from build123d import *

# Parameters (mm, degrees)
SPUR_START             = -44.074195703
SPUR_GEAR_AI_OUTLINE_R = 4.7625
SPUR_GEAR_AI_DEPTH     = 14.605
CUT_EXTRUDE1_DEPTH     = 39.307434666


# Read off the part's stored shape, not the designer's step: spur gear_ai
with BuildPart() as part:
    # spur gear_ai outline → spur gear_ai (new body)
    with BuildSketch(Plane.YZ.offset(SPUR_START)):
        with BuildLine():
            ThreePointArc((12.686684526, 14.250652999), (12.919777657, 14.586350288), (13.140720632, 14.930166051))
            ThreePointArc((13.140720632, 14.930166051), (12.265878987, 16.134593199), (11.016013995, 16.943190851))
            ThreePointArc((11.016013995, 16.943190851), (11.347770551, 17.651104248), (11.613753604, 18.386261921))
            ThreePointArc((11.613753604, 18.386261921), (13.069306498, 18.074238793), (14.539571561, 18.307290937))
            ThreePointArc((14.539571561, 18.307290937), (14.626455743, 18.70663567), (14.699007839, 19.108831233))
            ThreePointArc((14.699007839, 19.108831233), (13.429845234, 19.88678942), (11.965683625, 20.155533616))
            ThreePointArc((11.965683625, 20.155533616), (12.001279988, 20.936518051), (11.965683625, 21.717502486))
            ThreePointArc((11.965683625, 21.717502486), (13.429845234, 21.986246682), (14.699007839, 22.764204869))
            ThreePointArc((14.699007839, 22.764204869), (14.626455743, 23.166400432), (14.539571561, 23.565745165))
            ThreePointArc((14.539571561, 23.565745165), (13.069306498, 23.79879731), (11.613753604, 23.486774182))
            ThreePointArc((11.613753604, 23.486774182), (11.347770551, 24.221931855), (11.016013995, 24.929845251))
            ThreePointArc((11.016013995, 24.929845251), (12.265878987, 25.738442903), (13.140720632, 26.942870051))
            ThreePointArc((13.140720632, 26.942870051), (12.919777657, 27.286685815), (12.686684526, 27.622383104))
            ThreePointArc((12.686684526, 27.622383104), (11.239151532, 27.275049128), (10.013802086, 26.42976137))
            ThreePointArc((10.013802086, 26.42976137), (9.486733126, 27.007171189), (8.909323306, 27.534240149))
            ThreePointArc((8.909323306, 27.534240149), (9.754611065, 28.759589595), (10.10194504, 30.207122589))
            ThreePointArc((10.10194504, 30.207122589), (9.766247751, 30.44021572), (9.422431988, 30.661158695))
            ThreePointArc((9.422431988, 30.661158695), (8.21800484, 29.78631705), (7.409407188, 28.536452058))
            ThreePointArc((7.409407188, 28.536452058), (6.701493792, 28.868208614), (5.966336119, 29.134191667))
            ThreePointArc((5.966336119, 29.134191667), (6.278359246, 30.589744561), (6.045307102, 32.060009624))
            ThreePointArc((6.045307102, 32.060009624), (5.645962369, 32.146893806), (5.243766806, 32.219445902))
            ThreePointArc((5.243766806, 32.219445902), (4.465808619, 30.950283297), (4.197064423, 29.486121688))
            ThreePointArc((4.197064423, 29.486121688), (3.416079988, 29.521718051), (2.635095553, 29.486121688))
            ThreePointArc((2.635095553, 29.486121688), (2.366351357, 30.950283297), (1.58839317, 32.219445902))
            ThreePointArc((1.58839317, 32.219445902), (1.186197607, 32.146893806), (0.786852874, 32.060009624))
            ThreePointArc((0.786852874, 32.060009624), (0.55380073, 30.589744561), (0.865823857, 29.134191667))
            ThreePointArc((0.865823857, 29.134191667), (0.130666184, 28.868208614), (-0.577247212, 28.536452058))
            ThreePointArc((-0.577247212, 28.536452058), (-1.385844864, 29.78631705), (-2.590272012, 30.661158695))
            ThreePointArc((-2.590272012, 30.661158695), (-2.934087775, 30.44021572), (-3.269785064, 30.207122589))
            ThreePointArc((-3.269785064, 30.207122589), (-2.922451089, 28.759589595), (-2.07716333, 27.534240149))
            ThreePointArc((-2.07716333, 27.534240149), (-2.65457315, 27.007171189), (-3.18164211, 26.42976137))
            ThreePointArc((-3.18164211, 26.42976137), (-4.406991556, 27.275049128), (-5.85452455, 27.622383104))
            ThreePointArc((-5.85452455, 27.622383104), (-6.087617681, 27.286685815), (-6.308560656, 26.942870051))
            ThreePointArc((-6.308560656, 26.942870051), (-5.43371901, 25.738442903), (-4.183854019, 24.929845251))
            ThreePointArc((-4.183854019, 24.929845251), (-4.515610574, 24.221931855), (-4.781593628, 23.486774182))
            ThreePointArc((-4.781593628, 23.486774182), (-6.237146522, 23.79879731), (-7.707411585, 23.565745165))
            ThreePointArc((-7.707411585, 23.565745165), (-7.794295767, 23.166400432), (-7.866847863, 22.764204869))
            ThreePointArc((-7.866847863, 22.764204869), (-6.597685258, 21.986246682), (-5.133523649, 21.717502486))
            ThreePointArc((-5.133523649, 21.717502486), (-5.169120012, 20.936518051), (-5.133523649, 20.155533616))
            ThreePointArc((-5.133523649, 20.155533616), (-6.597685258, 19.88678942), (-7.866847863, 19.108831233))
            ThreePointArc((-7.866847863, 19.108831233), (-7.794295767, 18.70663567), (-7.707411585, 18.307290937))
            ThreePointArc((-7.707411585, 18.307290937), (-6.237146522, 18.074238793), (-4.781593628, 18.386261921))
            ThreePointArc((-4.781593628, 18.386261921), (-4.515610574, 17.651104248), (-4.183854019, 16.943190851))
            ThreePointArc((-4.183854019, 16.943190851), (-5.43371901, 16.134593199), (-6.308560656, 14.930166051))
            ThreePointArc((-6.308560656, 14.930166051), (-6.087617681, 14.586350288), (-5.85452455, 14.250652999))
            ThreePointArc((-5.85452455, 14.250652999), (-4.406991556, 14.597986974), (-3.18164211, 15.443274733))
            ThreePointArc((-3.18164211, 15.443274733), (-2.65457315, 14.865864913), (-2.07716333, 14.338795953))
            ThreePointArc((-2.07716333, 14.338795953), (-2.922451089, 13.113446507), (-3.269785064, 11.665913513))
            ThreePointArc((-3.269785064, 11.665913513), (-2.934087775, 11.432820383), (-2.590272012, 11.211877407))
            ThreePointArc((-2.590272012, 11.211877407), (-1.385844864, 12.086719053), (-0.577247212, 13.336584044))
            ThreePointArc((-0.577247212, 13.336584044), (0.130666184, 13.004827489), (0.865823857, 12.738844436))
            ThreePointArc((0.865823857, 12.738844436), (0.55380073, 11.283291542), (0.786852874, 9.813026478))
            ThreePointArc((0.786852874, 9.813026478), (1.186197607, 9.726142296), (1.58839317, 9.6535902))
            ThreePointArc((1.58839317, 9.6535902), (2.366351357, 10.922752805), (2.635095553, 12.386914414))
            ThreePointArc((2.635095553, 12.386914414), (3.416079988, 12.351318051), (4.197064423, 12.386914414))
            ThreePointArc((4.197064423, 12.386914414), (4.465808619, 10.922752805), (5.243766806, 9.6535902))
            ThreePointArc((5.243766806, 9.6535902), (5.645962369, 9.726142296), (6.045307102, 9.813026478))
            ThreePointArc((6.045307102, 9.813026478), (6.278359246, 11.283291542), (5.966336119, 12.738844436))
            ThreePointArc((5.966336119, 12.738844436), (6.701493792, 13.004827489), (7.409407188, 13.336584044))
            ThreePointArc((7.409407188, 13.336584044), (8.21800484, 12.086719053), (9.422431988, 11.211877407))
            ThreePointArc((9.422431988, 11.211877407), (9.766247751, 11.432820383), (10.10194504, 11.665913513))
            ThreePointArc((10.10194504, 11.665913513), (9.754611065, 13.113446507), (8.909323306, 14.338795953))
            ThreePointArc((8.909323306, 14.338795953), (9.486733126, 14.865864913), (10.013802086, 15.443274733))
            ThreePointArc((10.013802086, 15.443274733), (11.239151532, 14.597986974), (12.686684526, 14.250652999))
        make_face()
        with Locations((3.416079988, 20.936518051)):
            Circle(SPUR_GEAR_AI_OUTLINE_R, mode=Mode.SUBTRACT)
    extrude(amount=SPUR_GEAR_AI_DEPTH)

    # Sketch1 → Cut-Extrude1 (cut, through all)
    with BuildSketch(Plane(origin=(-29.469195703, 0, 0), x_dir=(0, 0, -1), z_dir=(1, 0, 0))):
        Polygon((-18.186887394, 8.178579988), (-23.686148708, 8.178579988), (-26.435779365, 3.416079988), (-23.686148708, -1.346420012), (-18.186887394, -1.346420012), (-15.437256737, 3.416079988), align=None)
    extrude(amount=-CUT_EXTRUDE1_DEPTH, mode=Mode.SUBTRACT)


solid = part.part
Geometry check sheet. Reference: the model listing, model coordinates, mm. A direction names the side the tool comes from. Give positions to 0.01 mm unless a question says otherwise; leave off trailing zeros. Order: outer loops, then holes, each group sorted by start corner. A loop starts at its lowest first (then second) coordinate and runs counter-clockwise, first axis right, second up. Notation, with made-up numbers: (-34, 81) - (16, 81) arc R38 cw to (16, 119) - close; hole circle Ø1 at (81.5, 82). An arc over 180 degrees is marked (long way). Answer as a JSON object with one key per item and string values.
(1) Cross-section at C-C (y = 8.5). Record the cut outline in (x, z).
Report:
{"outline": "(-44.07, 11.82) - (-29.47, 11.82) - (-29.47, 30.06) - (-44.07, 30.06) - close"}
(2) Depth check by flat-ended pin: pin 1 Ø3 at (x, z) = (-39, 12) entering from +Y; pin 2 Ø1 at (x, z) = (-31, 29.5) entering from -Y; pin 3 Ø8 at (x, z) = (-38.5, 13) entering from -Y. Enter the tip coordinate at first touch or a pass-through.
Report:
{"pin 1": "y = 10.1", "pin 2": "y = -3.25", "pin 3": "y = -6.31"}
(3) Cross-section at A-A (z = 16.5). Record the cut outline in (x, y).
Report:
{"outline": "(-44.07, -4.99) - (-29.47, -4.99) - (-29.47, 1.58) - (-44.07, 1.58) - close; (-44.07, 5.26) - (-29.47, 5.26) - (-29.47, 11.82) - (-44.07, 11.82) - close"}
(4) Cross-section at B-B (y = 4.75). Record the cut outline in (x, z), then the cut area to 3 significant figures.
Report:
{"outline": "(-44.07, 10.33) - (-29.47, 10.33) - (-29.47, 16.21) - (-44.07, 16.21) - close; (-44.07, 25.67) - (-29.47, 25.67) - (-29.47, 31.54) - (-44.07, 31.54) - close", "area": "172 mm^2"}
(5) Tool access check on faces 4 (the cylindrical face through (-36.874, 11.352, 24.212)), 5 (the cylindrical face through (-36.874, 14.628, 23.161)), 6 (the cylindrical face through (-36.9, 12.3, 16.1)). Record the directions out of +Z, -Z, +X, -X, +Y, -Y that give a thin tool (end or side, any length) a straight path to the whole face; none if there is none.
Report:
{"face 4": "+X, -X", "face 5": "+Z, +X, -X, +Y", "face 6": "+X, -X, +Y"}
(6) Material ranges on line 1 (Y direction, x = -37.5, z = 21.25); line 2 (Y direction, x = -38.5, z = 13.25); line 3 (Z direction, x = -38.25, y = 12.25), recorded low to high.
Report:
{"line 1": "-5.16 to -1.35, 8.18 to 12", "line 2": "-2.86 to -0.61, -0.41 to 7.24, 7.45 to 9.69", "line 3": "14.3 to 16.15, 18.18 to 20.15, 21.73 to 23.69, 25.72 to 27.58"}
(7) Draft check along Y on faces 1 (the cylindrical face through (-36.874, 5.64, 9.725)), 2 (the cylindrical face through (-36.874, 1.181, 9.727)), 3 (the cylindrical face through (-36.9, 13.1, 23.8)). Enter one of: released by +Y, released by -Y, zero draft, split by the parting line, or undercut.
Report:
{"face 1": "released by +Y", "face 2": "released by -Y", "face 3": "undercut"}
